from build123d import *

# Parameters (mm, degrees)
CROQUIS1_R              = 25
CROQUIS1_R_2            = 4.7625
SALIENTE_EXTRUIR1_DEPTH = 3
CROQUIS2_R              = 2
CORTAR_EXTRUIR1_DEPTH   = 4
CROQUIS3_R              = 13.1125
CROQUIS3_R_2            = 11.1125
SALIENTE_EXTRUIR2_DEPTH = 4.5
CROQUIS3_2_R            = 11.1125
CROQUIS3_2_R_2          = 4.7625
CORTAR_EXTRUIR2_DEPTH   = 4


with BuildPart() as part:
    # Croquis1 → Saliente-Extruir1 (new body)
    with BuildSketch(Plane(origin=(0, 0, 0), x_dir=(1, 0, 0), z_dir=(0, 1, 0))):
        Circle(CROQUIS1_R)
        Circle(CROQUIS1_R_2, mode=Mode.SUBTRACT)
    extrude(amount=SALIENTE_EXTRUIR1_DEPTH)

    # Croquis2 → Cortar-Extruir1 (cut, through all)
    with BuildSketch(Plane(origin=(0, 3, 0), x_dir=(1, 0, 0), z_dir=(0, 1, 0))):
        with Locations((0, 17)):
            Circle(CROQUIS2_R)
        with Locations((14.722431864, 8.5)):
            Circle(CROQUIS2_R)
        with Locations((14.722431864, -8.5)):
            Circle(CROQUIS2_R)
        with Locations((0, -17)):
            Circle(CROQUIS2_R)
        with Locations((-14.722431864, -8.5)):
            Circle(CROQUIS2_R)
        with Locations((-14.722431864, 8.5)):
            Circle(CROQUIS2_R)
    extrude(amount=-CORTAR_EXTRUIR1_DEPTH, mode=Mode.SUBTRACT)

    # Croquis3 → Saliente-Extruir2 (add)
    with BuildSketch(Plane(origin=(0, 3, 0), x_dir=(1, 0, 0), z_dir=(0, 1, 0))):
        Circle(CROQUIS3_R)
        Circle(CROQUIS3_R_2, mode=Mode.SUBTRACT)
    extrude(amount=SALIENTE_EXTRUIR2_DEPTH)

    # Croquis3<2> → Cortar-Extruir2 (cut, through all)
    with BuildSketch(Plane(origin=(0, 3, 0), x_dir=(1, 0, 0), z_dir=(0, 1, 0))):
        Circle(CROQUIS3_2_R)
        Circle(CROQUIS3_2_R_2, mode=Mode.SUBTRACT)
    extrude(amount=-CORTAR_EXTRUIR2_DEPTH, mode=Mode.SUBTRACT)


solid = part.part
CAD build for the part. Positions are in the model's coordinates, mm. A direction names the side the tool comes from. Coordinates: 2 decimals unless noted, no trailing zeros. Loops run counter-clockwise (first coordinate to the right, second up) from the corner with the lowest first, then second, coordinate; pieces in that order, holes last. Notation, with made-up numbers: (-16, 64) - (4, 64) arc R9 ccw to (4, 70) - close; hole circle Ø1 at (88.5, 23.5). An arc over 180 degrees is marked (long way). Use one line per item in the form item = value. Start each with the question number.
1) Flat gauge pins, fed straight in: pin 1 (8 mm diameter, centred on x = 12.5, z = 1, fed in from -Y); pin 2 (2.5 mm diameter, centred on x = -14.72, z = -8.5, fed in from +Y); pin 3 (3 mm diameter, centred on x = -16.5, z = -18.5, fed in from +Y). Where does each tip first touch, or does it go through?
2) Band-saw the part on D-D (z = 8.5). Give the cut face in (x, y), and give its area (3 significant figures).
3) Drill centre lines: L1, parallel to Z at x = 0, y = 1.1; L2, parallel to X at y = 2.1, z = -8.5; L3, parallel to Y at x = 6.5, z = -21.5. Where is each one in solid material? Low to high. Write a range as from..to.
4) Two-plate mould, pull along X, no slides. Class faces 1 (the face through (0, 2, -19)), 2 (the face through (-16.2, 1.52, 7.15)), 3 (the face through (23.846, 1.479, -7.509)), 4 (the face through (-11, 7.5, -3)): +X half, -X half, draft (parallel to the pull), parting line (faces both ways), or undercut.
5) Band-saw the part on B-B (z = 3). Give the cut face in (x, y), and give its area (3 significant figures).
6) Tool access for faces 5 (the face through (-2.84, 5.22, 12.8)), 6 (the face through (0, 2, 15)): list every direction of +Z, -Z, +X, -X, +Y, -Y with a clear straight run to the whole face (end or side of a thin tool).
7) Band-saw the part on C-C (x = 5). Give the cut face in (y, z).
8) Band-saw the part on A-A (x = 0). Give the cut face in (y, z), and give its area (3 significant figures).
Check values:
q1.pin_1 = 0
q1.pin_2 = through
q1.pin_3 = 3
q2.outline = (-23.51, 0) - (-16.72, 0) - (-16.72, 3) - (-23.51, 3) - close; (-12.72, 0) - (-7.16, 0) - (-7.16, 7.5) - (-9.98, 7.5) - (-9.98, 3) - (-12.72, 3) - close; (7.16, 0) - (12.72, 0) - (12.72, 3) - (9.98, 3) - (9.98, 7.5) - (7.16, 7.5) - close; (16.72, 0) - (23.51, 0) - (23.51, 3) - (16.72, 3) - close
q2.area = 99.6 mm2
q3.L1 = -25..-19, -15..-11.11, 11.11..15, 19..25
q3.L2 = -23.51..-16.72, -12.72..-7.16, 7.16..12.72, 16.72..23.51
q3.L3 = 0..3
q4.face_1 = undercut
q4.face_2 = undercut
q4.face_3 = parting line
q4.face_4 = draft
q5.outline = (-24.82, 0) - (-10.7, 0) - (-10.7, 7.5) - (-12.76, 7.5) - (-12.76, 3) - (-24.82, 3) - close; (10.7, 0) - (24.82, 0) - (24.82, 3) - (12.76, 3) - (12.76, 7.5) - (10.7, 7.5) - close
q5.area = 103 mm2
q6.face_5 = +Y
q6.face_6 = +Y, -Y
q7.outline = (0, -24.49) - (3, -24.49) - (3, -12.12) - (7.5, -12.12) - (7.5, -9.92) - (0, -9.92) - close; (0, 9.92) - (7.5, 9.92) - (7.5, 12.12) - (3, 12.12) - (3, 24.49) - (0, 24.49) - close
q8.outline = (0, -25) - (3, -25) - (3, -19) - (0, -19) - close; (0, -15) - (3, -15) - (3, -13.11) - (7.5, -13.11) - (7.5, -11.11) - (0, -11.11) - close; (0, 11.11) - (7.5, 11.11) - (7.5, 13.11) - (3, 13.11) - (3, 15) - (0, 15) - close; (0, 19) - (3, 19) - (3, 25) - (0, 25) - close
q8.area = 77.3 mm2
